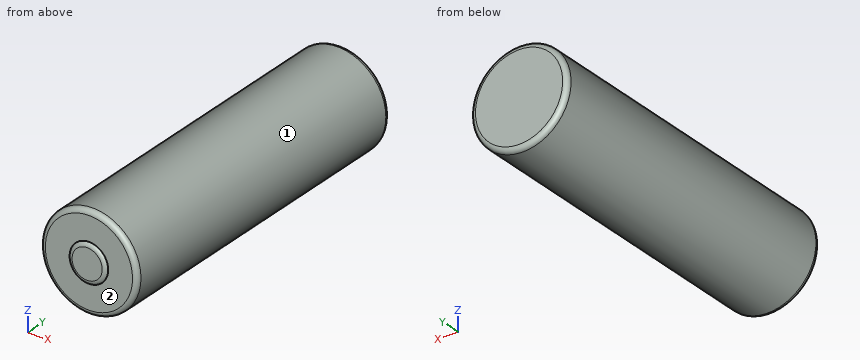
```python
from build123d import *

# Parameters (mm, degrees)
F0_R     = 10
F1_DEPTH = 70
F2_R     = 1
F3_R     = 3.9775912989
F4_DEPTH = 0.5


# Not quite as in the source:
# - a fillet or chamfer that OpenCascade refuses, or shapes differently, is made with other operations: its cross-section is extruded or revolved along the edge and cut away or added


with BuildPart() as f1:
    # F0 (on Front) → F1 (new body)
    with BuildSketch(Plane.XZ):
        Circle(F0_R)
    extrude(amount=F1_DEPTH)

    # F2
    f2_edges = [f1.edges().sort_by_distance(p)[0] for p in [
        (-10, -70, 0),
        (-10, 0, 0),
    ]]
    fillet(f2_edges, radius=F2_R)

    # F3 (on face) → F4 (join)
    with BuildSketch(Plane.XZ.offset(70)):
        Circle(F3_R)
    extrude(amount=F4_DEPTH)

    # F5: fillet of radius 1 on 1 edges, made by hand

    # F5_s1 → F5_t2 (revolve, cut)
    with BuildSketch(Plane.XY):
        with BuildLine():
            ThreePointArc((3.9775912989, -70), (3.6115658951, -70.3660254038), (3.1115658951, -70.5))
            Line((3.1115658951, -70.5), (3.9775912989, -70.5))
            Line((3.9775912989, -70.5), (3.9775912989, -70))
        make_face()
    revolve(axis=Axis((0, -70.5, 0), (0, -1, 0)), mode=Mode.SUBTRACT)


solid = f1.part
```
For this review, take the finished solid that the model builds, in its own axes (mm). Face numbers are marked on the shaded views. A direction names the side the tool comes from. Round coordinates to 2 decimals unless told otherwise and drop trailing zeros. Write each loop counter-clockwise with the first axis right and the second up, starting at its lowest first coordinate (ties: lowest second). Pieces come first, ordered by that corner, then holes. Notation, with made-up numbers: (-16.5, -21.75) - (-5.5, -21.75) arc R19 cw to (-5.5, -14.75) - close; hole circle Ø8 at (8.25, 59). An arc over 180 degrees is marked (long way). Answer as a JSON object with one key per item and string values.
1. Tool access review of the marked faces 1 and 2: name each direction out of +Z, -Z, +X, -X, +Y, -Y from which nothing blocks a thin tool from reaching the whole face with its end or side.
Response values:
{"face 1": "+Y, -Y", "face 2": "-Y"}
2. We need section A-A on y = -28. Give the boundary of the cut face in (x, z).
Response values:
{"outline": "circle Ø20 at (0, 0)"}
3. To check wall thickness, follow line 1 along Y through (x, z) = (8.5, -2.25); line 2 along X through (y, z) = (-13, -0.25); line 3 along X through (y, z) = (-18, 6.5). State the ranges of each line that lie inside material, in increasing order.
Response values:
{"line 1": "y = -70 to 0", "line 2": "x = -10 to 10", "line 3": "x = -7.6 to 7.6"}
4. For pin 1 Ø1.5 at (y, z) = (-56, 3.5) entering from -X; pin 2 Ø6 at (x, y) = (-4, -28) entering from -Z; pin 3 Ø8 at (y, z) = (-53.5, 6.5) entering from -X, all flat-tipped, find the tip position at first contact; note any pin that passes through.
Response values:
{"pin 1": "stops at x = -9.61", "pin 2": "stops at z = -9.95", "pin 3": "stops at x = -9.68"}
